Can you work these out from the model? Positions are in its coordinate system, mm. A direction names the side the tool comes from. Coordinates: 2 decimals unless noted, no trailing zeros. Order: outer loops, then holes, each group sorted by start corner. A loop starts at its lowest first (then second) coordinate and runs counter-clockwise, first axis right, second up. Notation, with made-up numbers: (-16, -37.5) -> (39, -37.5) arc R26 cw to (39, -5.5) -> close; hole circle Ø2 at (7.5, 63). An arc over 180 degrees is marked (long way). Answer in a Markdown table with one row per item.
```python
from build123d import *

# Parameters (mm, degrees)
SKETCH1_W           = 205.74
SKETCH1_H           = 88.9
BOSS_EXTRUDE1_DEPTH = 8.9916
SKETCH2_W           = 2.54
SKETCH2_H           = 44.45
CUT_EXTRUDE1_DEPTH  = 8.9916
CUT_EXTRUDE3_DEPTH  = 3.81


with BuildPart() as part:
    # Sketch1 → Boss-Extrude1 (new body)
    with BuildSketch(Plane.XY):
        Rectangle(SKETCH1_W, SKETCH1_H)
    extrude(amount=BOSS_EXTRUDE1_DEPTH)

    # Sketch2 → Cut-Extrude1 (cut)
    with BuildSketch(Plane.XY.offset(8.9916)):
        with Locations((0, -22.225)):
            Rectangle(SKETCH2_W, SKETCH2_H)
    extrude(amount=-CUT_EXTRUDE1_DEPTH, mode=Mode.SUBTRACT)

    # Sketch4 → Cut-Extrude3 (cut)
    with BuildSketch(Plane.XY.offset(8.9916)):
        with BuildLine():
            Line((-200.384333518, -4.590586805), (-4.804333518, -39.076617692))
            ThreePointArc((-4.804333518, -39.076617692), (-3.516617692, -40.915666482), (-5.355666482, -42.203382308))
            Line((-5.355666482, -42.203382308), (-200.935666482, -7.717351421))
            ThreePointArc((-200.935666482, -7.717351421), (-202.223382308, -5.878302631), (-200.384333518, -4.590586805))
        make_face()
        with BuildLine():
            Line((200.384333518, -4.590586805), (4.804333518, -39.076617692))
            ThreePointArc((4.804333518, -39.076617692), (3.516617692, -40.915666482), (5.355666482, -42.203382308))
            Line((5.355666482, -42.203382308), (200.935666482, -7.717351421))
            ThreePointArc((200.935666482, -7.717351421), (202.223382308, -5.878302631), (200.384333518, -4.590586805))
        make_face()
    extrude(amount=-CUT_EXTRUDE3_DEPTH, mode=Mode.SUBTRACT)


solid = part.part
```
(1) I need wall thicknesses on line 1 (X direction, y = -8, z = 1.5); line 2 (Y direction, x = -82, z = 7.25); line 3 (Y direction, x = -51, z = 8.75). Which ranges of each line are inside material? Lowest first, please. Write a range as [from, to].
Response values:
| item | result |
|---|---|
| line 1 | [-102.87, -1.27], [1.27, 102.87] |
| line 2 | [-44.45, -28.69], [-25.46, 44.45] |
| line 3 | [-44.45, -34.16], [-30.93, 44.45] |
(2) Suppose I cut it at A-A (x = 16). Please give me the cut outline in (y, z), and give its area (3 significant figures).
Response values:
| item | result |
|---|---|
| outline | (-44.45, 0) -> (44.45, 0) -> (44.45, 8.99) -> (-37.1, 8.99) -> (-37.1, 5.18) -> (-40.33, 5.18) -> (-40.33, 8.99) -> (-44.45, 8.99) -> close |
| area | 787 mm2 |
(3) We'd pull the mould along Y, two halves only. Please class faces 1 (the flat face through (53, -32, 5.182)), 2 (the flat face through (-1, 44.45, 4)), 3 (the flat face through (-1, 1, 0)), 4 (the flat face through (-54.52, -30.31, 7.11)): +Y half, -Y half, draft (parallel to the pull), parting line (faces both ways), or undercut.
Response values:
| item | result |
|---|---|
| face 1 | undercut |
| face 2 | +Y half |
| face 3 | draft |
| face 4 | undercut |
(4) On a 3-axis mill with a long thin cutter (end or side, diameter ignored), from which of +Z, -Z, +X, -X, +Y, -Y can I reach the whole of each face in a straight line? I mean faces 5 (the flat face through (54.52, -30.31, 7.11)), 6 (the flat face through (1.27, -23, 5)), 7 (the flat face through (-1, 1, 8.992)). Say none if no direction works.
Response values:
| item | result |
|---|---|
| face 5 | +Z |
| face 6 | +Z, -Z, -Y |
| face 7 | +Z, +X, -X, +Y, -Y |
